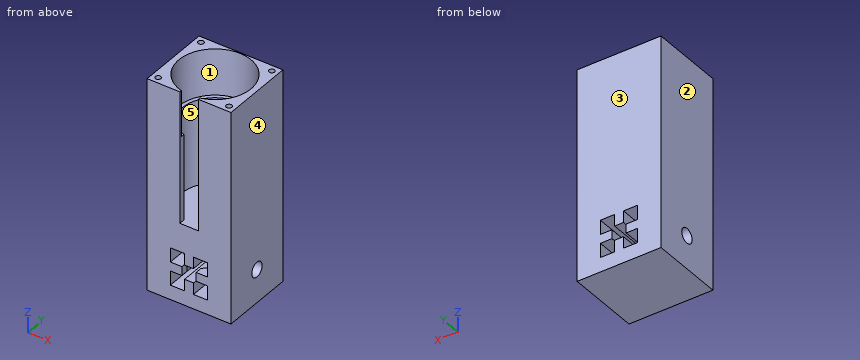
from build123d import *

# Parameters (mm, degrees)
BOSS_EXTRU_1_START                                = -20
BOSS_EXTRU_1_DEPTH                                = 40
ESQUISSE6_W                                       = 20.2
ESQUISSE6_H                                       = 20
ENL_V_MAT_EXTRU_1_DEPTH                           = 3
ESQUISSE14_W                                      = 30.8
ESQUISSE14_H                                      = 2.5
BOSS_EXTRU_3_DEPTH                                = 40
CHANFREIN1_SIZE                                   = 6.25
BOSS_EXTRU_4_DEPTH                                = 40
ESQUISSE21_W                                      = 45.3
ESQUISSE21_H                                      = 40
BOSS_EXTRU_5_DEPTH                                = 81.15
ESQUISSE22_R                                      = 17.5
ENL_V_MAT_EXTRU_2_DEPTH                           = 71.15
ESQUISSE23_W                                      = 10
ESQUISSE23_H                                      = 71.15
ENL_V_MAT_EXTRU_6_DEPTH                           = 6.15
ESQUISSE24_R                                      = 19.5
ENL_V_MAT_EXTRU_7_DEPTH                           = 25
ESQUISSE25_W                                      = 33.3
ESQUISSE25_H                                      = 40
BOSS_EXTRU_6_DEPTH                                = 7.25
CHAMBRAGE_POUR_VIS_SIX_PANS_CREUX_M42_D           = 4.5
CHAMBRAGE_POUR_VIS_SIX_PANS_CREUX_M42_DEPTH       = 12.55
CHAMBRAGE_POUR_VIS_SIX_PANS_CREUX_M42_CBORE_D     = 8
CHAMBRAGE_POUR_VIS_SIX_PANS_CREUX_M42_CBORE_DEPTH = 8.25
ESQUISSE28_W                                      = 33.3
ESQUISSE28_H                                      = 40
BOSS_EXTRU_7_DEPTH                                = 7.25
CHAMBRAGE_POUR_VIS_SIX_PANS_CREUX_M43_D           = 4.5
CHAMBRAGE_POUR_VIS_SIX_PANS_CREUX_M43_CBORE_D     = 8
CHAMBRAGE_POUR_VIS_SIX_PANS_CREUX_M43_CBORE_DEPTH = 8.25
ESQUISSE34_R                                      = 1.5
ENL_V_MAT_EXTRU_8_DEPTH                           = 15


# Read off the part's stored shape, not the designer's step: Boss.-Extru.1
with BuildPart() as part:
    # Boss.-Extru.1 outline → Boss.-Extru.1 (new body)
    with BuildSketch(Plane(origin=(0, 0, 0), x_dir=(1, 0, 0), z_dir=(0, 1, 0)).offset(BOSS_EXTRU_1_START)):
        Polygon((-10.1, -2.4), (-3.85, -2.4), (-3.85, 2.4), (-10.1, 2.4), (-10.1, 10.1), (-2.4, 10.1), (-2.4, 3.85), (2.4, 3.85), (2.4, 10.1), (10.1, 10.1), (10.1, 2.4), (3.85, 2.4), (3.85, -2.4), (10.1, -2.4), (10.1, -15.4), (15.4, -15.4), (15.4, 15.4), (-15.4, 15.4), (-15.4, -15.4), (-10.1, -15.4), align=None)
    extrude(amount=BOSS_EXTRU_1_DEPTH)

    # Esquisse6 → Enlèv. mat.-Extru.1 (cut, symmetric)
    with BuildSketch(Plane.XY):
        Rectangle(ESQUISSE6_W, ESQUISSE6_H)
    extrude(amount=ENL_V_MAT_EXTRU_1_DEPTH, both=True, mode=Mode.SUBTRACT)

    # Esquisse14 → Boss.-Extru.3 (add)
    with BuildSketch(Plane.XZ.offset(20)):
        with Locations((0, -16.65)):
            Rectangle(ESQUISSE14_W, ESQUISSE14_H)
    extrude(amount=-BOSS_EXTRU_3_DEPTH)

    # Chanfrein1
    chanfrein1_edges = [part.edges().sort_by_distance(p)[0] for p in [
        (3.85, -10, 0),
        (-3.85, -10, 0),
    ]]
    chamfer(chanfrein1_edges, length=CHANFREIN1_SIZE - 0.0001)  # a hair under: the kernel refuses the full size

    # Esquisse20 → Boss.-Extru.4 (add)
    with BuildSketch(Plane(origin=(0, 20, 0), x_dir=(1, 0, 0), z_dir=(0, 1, 0))):
        Polygon((-10.1, -15.4), (10.1, -15.4), (10.1, -10.097741972), (2.4, -10.097741972), (2.4, -3.847741972), (-2.4, -3.847741972), (-2.4, -10.097741972), (-10.1, -10.097741972), align=None)
    extrude(amount=-BOSS_EXTRU_4_DEPTH)

    # Esquisse21 → Boss.-Extru.5 (add)
    with BuildSketch(Plane.XY.offset(15.4)):
        Rectangle(ESQUISSE21_W, ESQUISSE21_H)
    extrude(amount=BOSS_EXTRU_5_DEPTH)

    # Esquisse22 → Enlèv. mat.-Extru.2 (cut)
    with BuildSketch(Plane.XY.offset(96.55)):
        Circle(ESQUISSE22_R)
    extrude(amount=-ENL_V_MAT_EXTRU_2_DEPTH, mode=Mode.SUBTRACT)

    # Esquisse23 → Enlèv. mat.-Extru.6 (cut)
    with BuildSketch(Plane(origin=(0, -20, 0), x_dir=(-1, 0, 0), z_dir=(0, -1, 0))):
        with Locations((0, -60.975)):
            Rectangle(ESQUISSE23_W, ESQUISSE23_H)
    extrude(amount=-ENL_V_MAT_EXTRU_6_DEPTH, mode=Mode.SUBTRACT)

    # Esquisse24 → Enlèv. mat.-Extru.7 (cut)
    with BuildSketch(Plane.XY.offset(96.55)):
        Circle(ESQUISSE24_R)
    extrude(amount=-ENL_V_MAT_EXTRU_7_DEPTH, mode=Mode.SUBTRACT)

    # Esquisse25 → Boss.-Extru.6 (add)
    with BuildSketch(Plane(origin=(15.4, 0, 0), x_dir=(0, 0, -1), z_dir=(1, 0, 0))):
        with Locations((1.25, 0)):
            Rectangle(ESQUISSE25_W, ESQUISSE25_H)
    extrude(amount=BOSS_EXTRU_6_DEPTH)

    # Chambrage pour vis à six pans creux M42
    with Locations(Plane(origin=(22.65, 0, 0), x_dir=(0, 0, -1), z_dir=(1, 0, 0))):
        with Locations((0, 0)):
            CounterBoreHole(CHAMBRAGE_POUR_VIS_SIX_PANS_CREUX_M42_D / 2, CHAMBRAGE_POUR_VIS_SIX_PANS_CREUX_M42_CBORE_D / 2, CHAMBRAGE_POUR_VIS_SIX_PANS_CREUX_M42_CBORE_DEPTH, depth=CHAMBRAGE_POUR_VIS_SIX_PANS_CREUX_M42_DEPTH)

    # Esquisse28 → Boss.-Extru.7 (add)
    with BuildSketch(Plane.ZY.offset(15.4)):
        with Locations((-1.25, 0)):
            Rectangle(ESQUISSE28_W, ESQUISSE28_H)
    extrude(amount=BOSS_EXTRU_7_DEPTH)

    # Chambrage pour vis à six pans creux M43 (through all)
    with Locations(Plane.ZY.offset(22.65)):
        with Locations((0, 0)):
            CounterBoreHole(CHAMBRAGE_POUR_VIS_SIX_PANS_CREUX_M43_D / 2, CHAMBRAGE_POUR_VIS_SIX_PANS_CREUX_M43_CBORE_D / 2, CHAMBRAGE_POUR_VIS_SIX_PANS_CREUX_M43_CBORE_DEPTH)

    # Esquisse34 → Enlèv. mat.-Extru.8 (cut)
    with BuildSketch(Plane.XY.offset(96.55)):
        with Locations((-19.15, 16.5)):
            Circle(ESQUISSE34_R)
        with Locations((-19.15, -16.5)):
            Circle(ESQUISSE34_R)
        with Locations((19.15, 16.5)):
            Circle(ESQUISSE34_R)
        with Locations((19.15, -16.5)):
            Circle(ESQUISSE34_R)
    extrude(amount=-ENL_V_MAT_EXTRU_8_DEPTH, mode=Mode.SUBTRACT)


solid = part.part
The listing builds one solid part. Answer for the finished solid, in the listing's coordinates (mm). Face numbers are marked on the shaded views. A direction names the side the tool comes from. Give positions to 0.01 mm unless a question says otherwise; leave off trailing zeros. Loops run counter-clockwise (first coordinate to the right, second up) from the corner with the lowest first, then second, coordinate; pieces in that order, holes last.
Item 1: Each of these flat-tipped pins is pushed along its axis until it touches: pin 1 Ø4 at (x, y) = (-6.5, 1) entering from +Z; pin 2 Ø2 at (x, y) = (-17, 6) entering from +Z. Where does it stop, or does it pass through?
Derived:
pin 1: stops at z = 25.4
pin 2: stops at z = 71.55
Item 2: A cutting plane is placed at B-B (z = 86.5). Give the vertices of the cut face in (x, y), then the cut area to 3 significant figures.
Derived:
outline: (-22.65, -20) - (-5, -20) - (-5, -18.85) arc R19.5 cw (long way) to (5, -18.85) - (5, -20) - (22.65, -20) - (22.65, 20) - (-22.65, 20) - close; hole circle Ø3 at (-19.15, -16.5); hole circle Ø3 at (-19.15, 16.5); hole circle Ø3 at (19.15, -16.5); hole circle Ø3 at (19.15, 16.5)
area: 582 mm2
Item 3: A cutting plane is placed at A-A (x = 0). Give the vertices of the cut face in (y, z), then the cut area to 3 significant figures.
Derived:
outline: (-20, -17.9) - (20, -17.9) - (20, -3.85) - (-20, -3.85) - close; (-20, 3.85) - (20, 3.85) - (20, 96.55) - (19.5, 96.55) - (19.5, 71.55) - (17.5, 71.55) - (17.5, 25.4) - (-20, 25.4) - close
area: 1,550 mm2
Item 4: A tool of negligible diameter and unlimited length cuts with its end or side. For the marked faces 4 and 5, from which of +Z, -Z, +X, -X, +Y, -Y can it reach the whole face along a straight path? Write none if from no direction.
Derived:
face 4: +Z, -Z, +X, +Y, -Y
face 5: +Z
Item 5: A cutting plane is placed at C-C (x = 9). Give the vertices of the cut face in (y, z), then the cut area to 3 significant figures.
Derived:
outline: (-20, -17.9) - (20, -17.9) - (20, -10.1) - (-20, -10.1) - close; (-20, -2.4) - (-11.1, -2.4) - (-11.1, 2.4) - (-20, 2.4) - close; (-20, 10.1) - (20, 10.1) - (20, 96.55) - (17.3, 96.55) - (17.3, 71.55) - (15.01, 71.55) - (15.01, 25.4) - (-15.01, 25.4) - (-15.01, 71.55) - (-17.3, 71.55) - (-17.3, 96.55) - (-20, 96.55) - close; (10, -2.4) - (20, -2.4) - (20, 2.4) - (10, 2.4) - close
area: 1,610 mm2
Item 6: Find the intervals of material crossed by line 1 along Z through (x, y) = (-7.5, 11.5); line 2 along Y through (x, z) = (-17, 0); line 3 along Z through (x, y) = (-17, 1), in increasing order.
Derived:
line 1: z = -17.9 to -10.1, -2.4 to 2.4, 10.1 to 25.4
line 2: y = -20 to -4, 4 to 20
line 3: z = -17.9 to -3.87, 3.87 to 25.4
Item 7: A cutting plane is placed at D-D (z = 7). Give the vertices of the cut face in (x, y), then the cut area to 3 significant figures.
Derived:
outline: (-22.65, -20) - (-10.1, -20) - (-10.1, 20) - (-22.65, 20) - close; (-2.4, -20) - (2.4, -20) - (2.4, 20) - (-2.4, 20) - close; (10.1, -20) - (22.65, -20) - (22.65, 20) - (10.1, 20) - close
area: 1,200 mm2
Item 8: Determine the mould class of the marked faces 1, 2 and 3 for opening direction X: +X half, -X half, draft (parallel to the pull), parting line (faces both ways), or undercut.
Derived:
face 1: undercut
face 2: -X half
face 3: draft
